Check sheet for the drawn part. Datum: minimum x, y, z corner. Units: mm. A direction names the side the tool comes from. Round coordinates to 2 decimals unless told otherwise and drop trailing zeros. Order: outer loops, then holes, each group sorted by start corner. A loop starts at its lowest first (then second) coordinate and runs counter-clockwise, first axis right, second up.
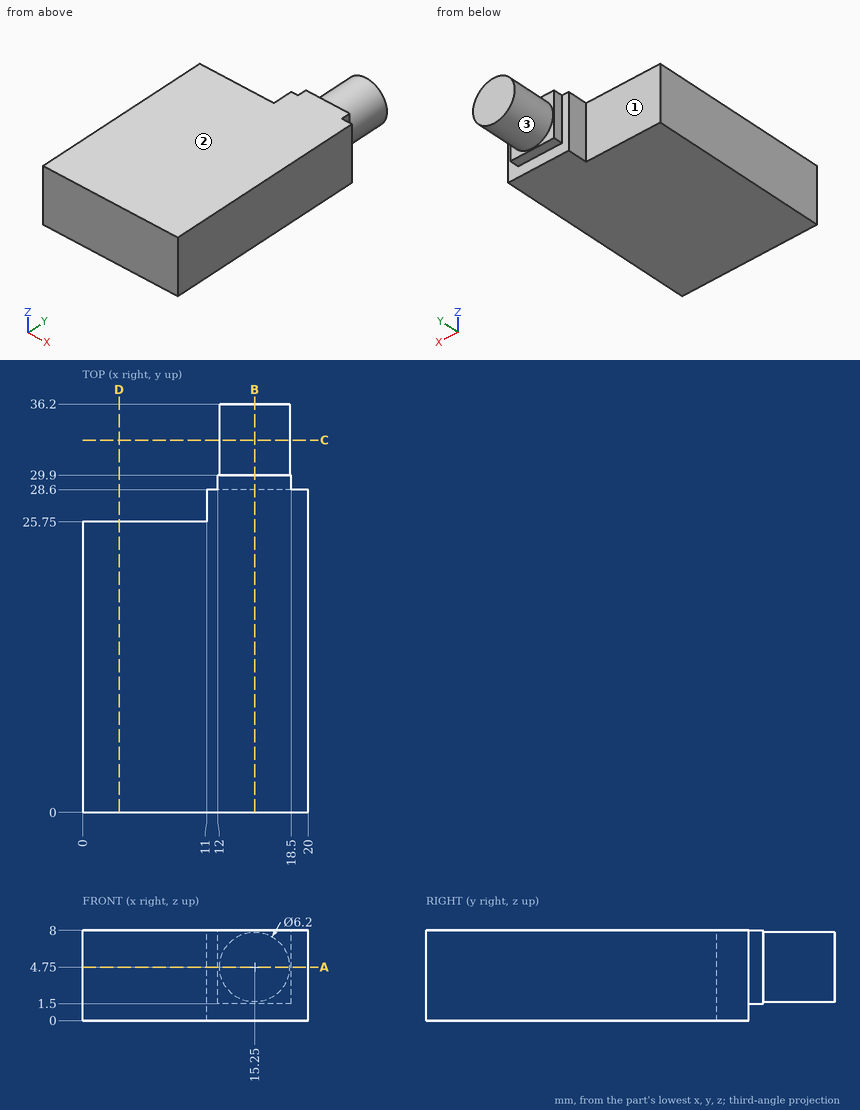
1) Set-up check for the marked faces 1, 2 and 3: record each of +Z, -Z, +X, -X, +Y, -Y from which the full face is reachable in a straight line by a thin tool's end or side.
2) Scan lines: line 1 (X direction, y = 27.5, z = 6.25); line 2 (Y direction, x = 6.5, z = 5.5); line 3 (X direction, y = 30.5, z = 3.5). Record each from-to range of solid material in increasing order.
3) Sectioned sample at A-A on z = 4.75. Record the cut outline in (x, y), and give its area (3 significant figures).
4) Sectioned sample at D-D on x = 3.25. Record the cut outline in (y, z).
5) Sectioned sample at B-B on x = 15.25. Record the cut outline in (y, z).
6) Gauge pin test, flat ends, axial feed: pin 1 (4 mm diameter, centred on y = 15.5, z = 6.5, fed in from -X); pin 2 (2.5 mm diameter, centred on x = 4, z = 3.5, fed in from +Y); pin 3 (1 mm diameter, centred on y = 29.5, z = 6, fed in from -X). Record the tip position at first contact, or that the pin passes through.
7) Sectioned sample at C-C on y = 33. Record the cut outline in (x, z), and give its area (3 significant figures).
Values found:
1. face 1: +Z, -Z, -X, +Y
1. face 2: +Z, +X, -X, +Y, -Y
1. face 3: +Y
2. line 1: x = 11 to 20
2. line 2: y = 0 to 25.75
2. line 3: x = 12.41 to 18.09
3. outline: (0, 0) - (20, 0) - (20, 28.6) - (18.5, 28.6) - (18.5, 29.9) - (18.35, 29.9) - (18.35, 36.2) - (12.15, 36.2) - (12.15, 29.9) - (12, 29.9) - (12, 28.6) - (11, 28.6) - (11, 25.75) - (0, 25.75) - close
3. area: 588 mm2
4. outline: (0, 0) - (25.75, 0) - (25.75, 8) - (0, 8) - close
5. outline: (0, 0) - (28.6, 0) - (28.6, 1.5) - (29.9, 1.5) - (29.9, 1.65) - (36.2, 1.65) - (36.2, 7.85) - (29.9, 7.85) - (29.9, 8) - (0, 8) - close
6. pin 1: stops at x = 0
6. pin 2: stops at y = 25.75
6. pin 3: stops at x = 12
7. outline: circle Ø6.2 at (15.25, 4.75)
7. area: 30.2 mm2
